Autodesk Fusion 360 part; units mm, degrees
sketch "Sketch1" plane through (0, 0, 0) normal (0, 1, 0) x (1, 0, 0)
  circle A0 centre (0, 0) radius 25
  line L0 (20, 0) -> (35, 0)
  line L1 (7.1429, -23.9579) -> (39.2857, -14.3747)
  line L2 (-2.1697, 26.7343) -> (39.2857, 14.3747)
  arc A1 (39.2857, -14.3747) -> (39.2857, 14.3747) centre (35, 0) ccw
  line L3 (0, -63.6354) -> (0, 71.5668)
  line L4 (-7.1429, -23.9579) -> (-39.2857, -14.3747)
  arc A2 (-39.2857, 14.3747) -> (-39.2857, -14.3747) centre (-35, 0) ccw
  line L5 (2.1697, 26.7343) -> (-39.2857, 14.3747)
  circle A3 centre (0, 0) radius 25
  circle A4 centre (-35, 0) radius 6
  circle A5 centre (35, 0) radius 6
  dimension "d1" = 50
  dimension "d2" = 35
  dimension "d3" = 30
  dimension "d4" = 12
  dimension "d5" = 12
extrude "Extrude1" add sketch "Sketch1" along normal blind 10 contours A0 L1 L2 A1 A3 | A0 L4 A2 L5 A3 makes body 1 at (31.6163, 0, 10.1046) makes body 2 at (-31.6163, 0, -10.1046)
sketch "Sketch2" plane through (0, 0, 0) normal (0, 1, 0) x (1, 0, 0)
  circle A0 centre (0, 0) radius 25
  circle A1 centre (0, 0) radius 25
  dimension "d8" = 50
  dimension "d9" = 50
extrude "Extrude2" add sketch "Sketch2" along normal blind 38 bodies 1 2
hole "Hole1" at (-0.4637, 38, 0.1546) direction (0, -1, 0) diameter 20 depth 38 tip angle 180 counterbore diameter 30 counterbore depth 6 bodies 1
sketch "Sketch3" plane through (0, 0, 0) normal (0, 0, 1) x (1, 0, 0)
  line L0 (0, 0) -> (0, 26)
  dimension "d17" = 26
hole "Hole2" at (0, 26, 0) direction (0, 0, -1) diameter 6 depth 25 tip angle 180 bodies 1
Geometry check sheet. Reference: the model listing, model coordinates, mm. A direction names the side the tool comes from. Give positions to 0.01 mm unless a question says otherwise; leave off trailing zeros. Write each loop counter-clockwise with the first axis right and the second up, starting at its lowest first coordinate (ties: lowest second). Pieces come first, ordered by that corner, then holes. Notation, with made-up numbers: (-1, 36.25) - (30, 36.25) arc R18 ccw to (30, 40.25) - close; hole circle Ø1 at (-36.75, -28.75). An arc over 180 degrees is marked (long way). Put each result on its own line as item: value.
1. Go/stop test with flat-tipped pins: pin 1 (8 mm diameter, centred on x = 36.5, y = 16, fed in from +Z); pin 2 (13 mm diameter, centred on x = 39, z = -2.5, fed in from +Y); pin 3 (9 mm diameter, centred on x = 0.5, z = 6, fed in from +Y); pin 4 (12 mm diameter, centred on x = 39, y = 6, fed in from +Z). Record where each tip stops, or that it passes through.
Ans:
pin 1: passes through
pin 2: stops at y = 10
pin 3: stops at y = 32
pin 4: stops at z = 16.25
2. Thickness scan on line 1 (X direction, y = 2.5, z = -2.5); line 2 (Z direction, x = 35, y = 7); line 3 (X direction, y = 8, z = -3). Record the ranges inside material, lowest first.
Ans:
line 1: x = -49.79 to -40.45, -29.55 to -10.1, 9.18 to 29.55, 40.45 to 49.79
line 2: z = -15.65 to -6, 6 to 15.65
line 3: x = -49.7 to -40.2, -29.8 to -9.95, 9.03 to 29.8, 40.2 to 49.7
3. Sectioned sample at D-D, the plane z = -20. Enter the section's corners in (x, y).
Ans:
outline: (-20.42, 0) - (20.42, 0) - (20.42, 10) - (15, 10) - (15, 38) - (-15, 38) - (-15, 10) - (-20.42, 10) - close; hole circle Ø6 at (0, 26)
4. Set-up check for faces 1 (the flat face through (-22.989, 4.93, -19.233)), 2 (the cylindrical face through (0, 29, -17)), 3 (the cylindrical face through (-24.976, 22.956, 1.099)): record each of +Z, -Z, +X, -X, +Y, -Y from which the full face is reachable in a straight line by a thin tool's end or side.
Ans:
face 1: -Z, -X, +Y, -Y
face 2: -Z
face 3: +Y
5. Sectioned sample at A-A, the plane z = 2.5. Enter the section's corners in (x, y), plus the area to 3 significant figures.
Ans:
outline: (-49.79, 0) - (-40.45, 0) - (-40.45, 10) - (-49.79, 10) - close; (-29.55, 0) - (-10.18, 0) - (-10.18, 32) - (-15.28, 32) - (-15.28, 38) - (-24.87, 38) - (-24.87, 10) - (-29.55, 10) - close; (9.26, 0) - (29.55, 0) - (29.55, 10) - (24.87, 10) - (24.87, 38) - (14.35, 38) - (14.35, 32) - (9.26, 32) - close; (40.45, 0) - (49.79, 0) - (49.79, 10) - (40.45, 10) - close
area: 1,370 mm²
6. Sectioned sample at C-C, the plane y = 8. Enter the section's corners in (x, z).
Ans:
outline: (-39.29, -14.37) - (-7.14, -23.96) arc R25 ccw to (7.14, -23.96) - (39.29, -14.37) arc R15 ccw to (39.29, 14.37) - (7.14, 23.96) arc R25 ccw to (-7.14, 23.96) - (-39.29, 14.37) arc R15 ccw to start; hole circle Ø12 at (-35, 0); hole circle Ø20 at (-0.46, 0.15); hole circle Ø12 at (35, 0)
7. Draft check along Z on faces 4 (the flat face through (11, 38, 11)), 5 (the cylindrical face through (-3.47, 15.78, 9.69)), 6 (the cylindrical face through (50, 5, 0)), 7 (the cylindrical face through (30.24, 4.93, -3.65)). Enter one of: +Z half, -Z half, draft (parallel to the pull), parting line (faces both ways), or undercut.
Ans:
face 4: draft
face 5: undercut
face 6: parting line
face 7: undercut
8. Sectioned sample at B-B, the plane x = -35. Enter the section's corners in (y, z), plus the area to 3 significant figures.
Ans:
outline: (0, -15.65) - (10, -15.65) - (10, -6) - (0, -6) - close; (0, 6) - (10, 6) - (10, 15.65) - (0, 15.65) - close
area: 193 mm²
